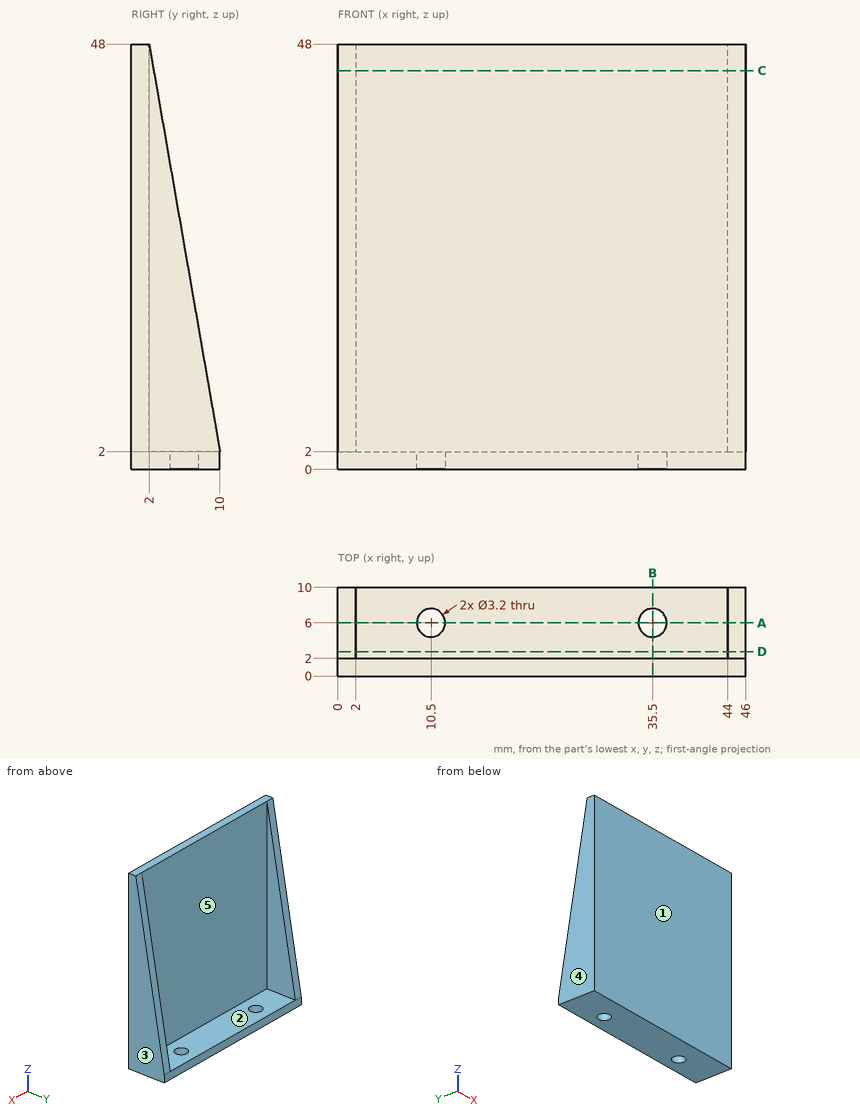
Design review of the part shown in the three views and the two pictorial views. Dimensions are in mm from the part's minimum x, y and z. A direction names the side the tool comes from. Coordinates: 2 decimals unless noted, no trailing zeros. Write each loop counter-clockwise with the first axis right and the second up, starting at its lowest first coordinate (ties: lowest second). Pieces come first, ordered by that corner, then holes.
1) We need section C-C on z = 45. State the section outline as (x, y) points, then the cut area to 3 significant figures.
2) We need section D-D on y = 2.75. State the section outline as (x, z) points.
3) Machinability: for the marked faces 1 and 2, which of the approach directions +Z, -Z, +X, -X, +Y, -Y give a long, thin tool a straight path to every point of the face, cutting with its end or side? Answer none if there is none.
4) We need section A-A on y = 6. State the section outline as (x, z) points.
5) The part is to be moulded in two halves that separate along X. For the marked faces 3, 4 and 5, say which applies: pulls with the +X half, pulls with the -X half, needs draft (parallel to the pull), parting line crosses it, or undercut.
6) Clearance check with flat-ended pins moving along their axes: pin 1 Ø5 at (x, y) = (35.5, 6) entering from +Z; pin 2 Ø12 at (x, z) = (29, 18) entering from +Y. State where each tip first meets the part, or that it passes through.
7) We need section B-B on x = 35.5. State the section outline as (y, z) points.
8) To check wall thickness, follow probe 1 along X at (y, z) = (4, 25); probe 2 along Y at (x, z) = (10.5, 0.85); probe 3 along Z at (x, y) = (17, 5). State the ranges of each line that lie inside material, in increasing order.
Answer list:
1. outline: (0, 0) - (46, 0) - (46, 2.52) - (44, 2.52) - (44, 2) - (2, 2) - (2, 2.52) - (0, 2.52) - close
1. area: 94.1 mm2
2. outline: (0, 0) - (46, 0) - (46, 43.69) - (44, 43.69) - (44, 2) - (2, 2) - (2, 43.69) - (0, 43.69) - close
3. face 1: +Z, -Z, +X, -X, -Y
3. face 2: +Z, +Y
4. outline: (0, 0) - (8.9, 0) - (8.9, 2) - (2, 2) - (2, 25) - (0, 25) - close; (12.1, 0) - (33.9, 0) - (33.9, 2) - (12.1, 2) - close; (37.1, 0) - (46, 0) - (46, 25) - (44, 25) - (44, 2) - (37.1, 2) - close
5. face 3: pulls with the +X half
5. face 4: pulls with the -X half
5. face 5: undercut
6. pin 1: stops at z = 2
6. pin 2: stops at y = 2
7. outline: (0, 0) - (4.4, 0) - (4.4, 2) - (2, 2) - (2, 48) - (0, 48) - close; (7.6, 0) - (10, 0) - (10, 2) - (7.6, 2) - close
8. probe 1: x = 0 to 2, 44 to 46
8. probe 2: y = 0 to 4.4, 7.6 to 10
8. probe 3: z = 0 to 2
